```python
from build123d import *

# Parameters (mm, degrees)
SALIENTE_EXTRUIR1_START = -80
CROQUIS1_W              = 13.5
CROQUIS1_H              = 13.5
CROQUIS1_W_2            = 11.5
CROQUIS1_H_2            = 11.5
SALIENTE_EXTRUIR1_DEPTH = 330


with BuildPart() as part:
    # Croquis1 → Saliente-Extruir1 (new body)
    with BuildSketch(Plane.XY.offset(SALIENTE_EXTRUIR1_START)):
        with Locations((0, 10.75)):
            Rectangle(CROQUIS1_W, CROQUIS1_H)
        with Locations((0, 10.75)):
            Rectangle(CROQUIS1_W_2, CROQUIS1_H_2, mode=Mode.SUBTRACT)
    extrude(amount=SALIENTE_EXTRUIR1_DEPTH)


solid = part.part
```
The model under review builds one solid part; all positions refer to its coordinate system, in mm. A direction names the side the tool comes from. Round coordinates to 2 decimals unless told otherwise and drop trailing zeros. Order: outer loops, then holes, each group sorted by start corner. A loop starts at its lowest first (then second) coordinate and runs counter-clockwise, first axis right, second up.
(1) For P1, Ø3, axis at x = -3.5, y = 14.5, coming from the -Z side, flat-tipped, find the tip position at first contact; note if it passes through.
Working result:
P1: passes through
(2) Wall thickness on L1, parallel to Y at x = 3.25, z = 81; L2, parallel to X at y = 13.5, z = -32.5: over which ranges is each line inside the solid? List them lowest first.
Working result:
L1: y = 4 to 5, 16.5 to 17.5
L2: x = -6.75 to -5.75, 5.75 to 6.75
(3) Mouldability with a two-part tool opening along Y and no side actions: class faces 3 (the face through (0, 17.5, 83)), 4 (the face through (-5.75, 11, 83)), 5 (the face through (-6.75, 11, 83)), 6 (the face through (0, 16.5, 83)) as released by +Y, released by -Y, zero draft, split by the parting line, or undercut.
Working result:
face 3: released by +Y
face 4: undercut
face 5: zero draft
face 6: undercut
(4) Tool access review of faces 1 (the face through (5.75, 11, 83)), 2 (the face through (0, 4, 83)): name each direction out of +Z, -Z, +X, -X, +Y, -Y from which nothing blocks a thin tool from reaching the whole face with its end or side.
Working result:
face 1: +Z, -Z
face 2: +Z, -Z, +X, -X, -Y
(5) Take a section at C-C, the plane z = 220.5. State the section outline as (x, y) points, plus the area to 3 significant figures.
Working result:
outline: (-6.75, 4) - (6.75, 4) - (6.75, 17.5) - (-6.75, 17.5) - close; hole (-5.75, 5) - (5.75, 5) - (5.75, 16.5) - (-5.75, 16.5) - close
area: 50.0 mm2
(6) Take a section at A-A, the plane x = 1.25. State the section outline as (y, z) points.
Working result:
outline: (4, -80) - (5, -80) - (5, 250) - (4, 250) - close; (16.5, -80) - (17.5, -80) - (17.5, 250) - (16.5, 250) - close
(7) Take a section at B-B, the plane y = 8.75. State the section outline as (x, z) points, plus the area to 3 significant figures.
Working result:
outline: (-6.75, -80) - (-5.75, -80) - (-5.75, 250) - (-6.75, 250) - close; (5.75, -80) - (6.75, -80) - (6.75, 250) - (5.75, 250) - close
area: 660 mm2
